Verification items for the finished model (mm, model axes). A direction names the side the tool comes from. Give positions to 0.01 mm unless a question says otherwise; leave off trailing zeros. Order: outer loops, then holes, each group sorted by start corner. A loop starts at its lowest first (then second) coordinate and runs counter-clockwise, first axis right, second up. Notation, with made-up numbers: (35.5, 33) - (59.5, 33) arc R25 ccw to (59.5, 53) - close; hole circle Ø11 at (-1, -29.75). An arc over 180 degrees is marked (long way). Answer as a JSON object with one key per item and string values. Group by question number.
(1) Section check C-C (x = 8). Record the boundary of the cut face in (y, z).
(2) Section check D-D (z = -53.5). Record the boundary of the cut face in (x, y).
(3) Access from +Z, -Z, +X, -X, +Y, -Y to the whole of each face (thin tool, end or side, straight path). Record for faces 4 (the face through (12.52, 58.52, -30.84)), 5 (the face through (32, 0, -30)), 6 (the face through (32, 30, -3)).
(4) Section check B-B (y = 32). Record the boundary of the cut face in (x, z), then the cut area to 3 significant figures.
(5) Depth check by flat-ended pin: pin 1 Ø3 at (x, z) = (24.01, -21.51) entering from -Y; pin 2 Ø5 at (x, z) = (40.99, -21.51) entering from +Y. Enter the tip coordinate at first touch or a pass-through.
(6) Mould release check, pull along X, two halves, no side actions. Record for faces 1 (the face through (24.94, 1.48, -40.26)), 2 (the face through (32.04, 0.57, -59.4)), 3 (the face through (0, 59, -30)): +X half, -X half, draft (parallel to the pull), parting line (faces both ways), or undercut.
(7) Section check A-A (z = -30). Record the boundary of the cut face in (x, y).
(8) Thickness scan on line 1 (Y direction, x = 13, z = -5.5); line 2 (Z direction, x = 25, y = 46); line 3 (Z direction, x = 55, y = 59). Record the ranges inside material, lowest first.
```python
from build123d import *

# Parameters (mm, degrees)
EXTRUDE_1_DEPTH     = 65
SKETCH_2_R          = 2.5
CUT_EXTRUDE_1_DEPTH = 61
SKETCH_3_R          = 7
CUT_EXTRUDE_2_DEPTH = 61
CUT_EXTRUDE_4_REACH = 62
SKETCH_7_R          = 2
CUT_EXTRUDE_5_REACH = 62
SKETCH_8_R          = 19


with BuildPart() as part:
    # 草图1 → 凸台-拉伸1 (new body)
    with BuildSketch(Plane(origin=(0, 0, 0), x_dir=(0, 0, -1), z_dir=(1, 0, 0))):
        with BuildLine():
            Line((60, 2), (60, 58))
            ThreePointArc((60, 58), (59.414213562, 59.414213562), (58, 60))
            Line((58, 60), (2, 60))
            ThreePointArc((2, 60), (0.585786438, 59.414213562), (0, 58))
            Line((0, 58), (0, 2))
            ThreePointArc((0, 2), (0.585786438, 0.585786438), (2, 0))
            Line((2, 0), (58, 0))
            ThreePointArc((58, 0), (59.414213562, 0.585786438), (60, 2))
        make_face()
        with BuildLine():
            Line((3, 5), (3, 55))
            ThreePointArc((3, 55), (3.585786438, 56.414213562), (5, 57))
            Line((5, 57), (55, 57))
            ThreePointArc((55, 57), (56.414213562, 56.414213562), (57, 55))
            Line((57, 55), (57, 5))
            ThreePointArc((57, 5), (56.414213562, 3.585786438), (55, 3))
            Line((55, 3), (5, 3))
            ThreePointArc((5, 3), (3.585786438, 3.585786438), (3, 5))
        make_face(mode=Mode.SUBTRACT)
    extrude(amount=EXTRUDE_1_DEPTH)

    # 草图2 → 切除-拉伸1 (cut, through all)
    with BuildSketch(Plane(origin=(0, 60, 0), x_dir=(1, 0, 0), z_dir=(0, 1, 0))):
        with Locations((8, 6.5)):
            Circle(SKETCH_2_R)
        with Locations((55, 6.5)):
            Circle(SKETCH_2_R)
        with Locations((55, 53.5)):
            Circle(SKETCH_2_R)
        with Locations((8, 53.5)):
            Circle(SKETCH_2_R)
    extrude(amount=-CUT_EXTRUDE_1_DEPTH, mode=Mode.SUBTRACT)

    # 草图3 → 切除-拉伸2 (cut, through all)
    with BuildSketch(Plane.XY):
        with Locations((52.5, 32)):
            Circle(SKETCH_3_R)
    extrude(amount=-CUT_EXTRUDE_2_DEPTH, mode=Mode.SUBTRACT)

    # 草图7 → 切除-拉伸4 (cut, up to next)
    with BuildSketch(Plane.XZ, mode=Mode.PRIVATE) as cut_extrude_4_sk1:
        with Locations((40.985281374, -38.485281374)):
            Circle(SKETCH_7_R)
    cut_extrude_4_tool1 = extrude(cut_extrude_4_sk1.sketch, amount=-CUT_EXTRUDE_4_REACH, mode=Mode.PRIVATE) & part.part
    add(cut_extrude_4_tool1.solids().sort_by_distance((40.985281, 0, -38.485281))[0], mode=Mode.SUBTRACT)
    # 草图7 → 切除-拉伸4 (cut, up to next)
    with BuildSketch(Plane.XZ, mode=Mode.PRIVATE) as cut_extrude_4_sk2:
        with Locations((24.014718626, -38.485281374)):
            Circle(SKETCH_7_R)
    cut_extrude_4_tool2 = extrude(cut_extrude_4_sk2.sketch, amount=-CUT_EXTRUDE_4_REACH, mode=Mode.PRIVATE) & part.part
    add(cut_extrude_4_tool2.solids().sort_by_distance((24.014719, 0, -38.485281))[0], mode=Mode.SUBTRACT)
    # 草图7 → 切除-拉伸4 (cut, up to next)
    with BuildSketch(Plane.XZ, mode=Mode.PRIVATE) as cut_extrude_4_sk3:
        with Locations((24.014718626, -21.514718626)):
            Circle(SKETCH_7_R)
    cut_extrude_4_tool3 = extrude(cut_extrude_4_sk3.sketch, amount=-CUT_EXTRUDE_4_REACH, mode=Mode.PRIVATE) & part.part
    add(cut_extrude_4_tool3.solids().sort_by_distance((24.014719, 0, -21.514719))[0], mode=Mode.SUBTRACT)
    # 草图7 → 切除-拉伸4 (cut, up to next)
    with BuildSketch(Plane.XZ, mode=Mode.PRIVATE) as cut_extrude_4_sk4:
        with Locations((40.985281374, -21.514718626)):
            Circle(SKETCH_7_R)
    cut_extrude_4_tool4 = extrude(cut_extrude_4_sk4.sketch, amount=-CUT_EXTRUDE_4_REACH, mode=Mode.PRIVATE) & part.part
    add(cut_extrude_4_tool4.solids().sort_by_distance((40.985281, 0, -21.514719))[0], mode=Mode.SUBTRACT)

    # 草图8 → 切除-拉伸5 (cut, up to next)
    with BuildSketch(Plane(origin=(0, 60, 0), x_dir=(1, 0, 0), z_dir=(0, 1, 0)), mode=Mode.PRIVATE) as cut_extrude_5_sk1:
        with Locations((31.5, 30)):
            Circle(SKETCH_8_R)
    cut_extrude_5_tool1 = extrude(cut_extrude_5_sk1.sketch, amount=-CUT_EXTRUDE_5_REACH, mode=Mode.PRIVATE) & part.part
    add(cut_extrude_5_tool1.solids().sort_by_distance((31.5, 60, -30))[0], mode=Mode.SUBTRACT)


solid = part.part
```
Solutions:
{
 "1": {"outline": "(0, -58) arc R2 ccw to (2, -60) - (58, -60) arc R2 ccw to (60, -58) - (60, -56) - (56.73, -56) arc R2 cw to (55, -57) - (5, -57) arc R2 cw to (3.27, -56) - (0, -56) - close; (0, -51) - (3, -51) - (3, -9) - (0, -9) - close; (0, -4) - (3.27, -4) arc R2 cw to (5, -3) - (55, -3) arc R2 cw to (56.73, -4) - (60, -4) - (60, -2) arc R2 ccw to (58, 0) - (2, 0) arc R2 ccw to (0, -2) - close; (57, -51) - (60, -51) - (60, -9) - (57, -9) - close"},
 "2": {"outline": "(0, 0) - (5.5, 0) - (5.5, 3) - (0, 3) - close; (0, 57) - (5.5, 57) - (5.5, 60) - (0, 60) - close; (10.5, 0) - (52.5, 0) - (52.5, 3) - (10.5, 3) - close; (10.5, 57) - (52.5, 57) - (52.5, 60) - (10.5, 60) - close; (57.5, 0) - (65, 0) - (65, 3) - (57.5, 3) - close; (57.5, 57) - (65, 57) - (65, 60) - (57.5, 60) - close"},
 "3": {"face 4": "+Y", "face 5": "+Z, -Z, +X, -X, -Y", "face 6": "+X, -X"},
 "4": {"outline": "(0, -60) - (45.5, -60) - (45.5, -57) - (0, -57) - close; (0, -3) - (45.5, -3) - (45.5, 0) - (0, 0) - close; (59.5, -60) - (65, -60) - (65, -57) - (59.5, -57) - close; (59.5, -3) - (65, -3) - (65, 0) - (59.5, 0) - close", "area": "306 mm2"},
 "5": {"pin 1": "passes through", "pin 2": "stops at y = 3"},
 "6": {"face 1": "undercut", "face 2": "draft", "face 3": "-X half"},
 "7": {"outline": "(0, 0) - (65, 0) - (65, 3) - (0, 3) - close; (0, 57) - (12.5, 57) - (12.5, 60) - (0, 60) - close; (50.5, 57) - (65, 57) - (65, 60) - (50.5, 60) - close"},
 "8": {"line 1": "y = 0 to 3, 57 to 60", "line 2": "z = -60 to -57, -3 to 0", "line 3": "z = -59.73 to -56, -51 to -9, -4 to -0.27"}
}
